from build123d import *

# Parameters (mm, degrees)
SALIENTE_EXTRUIR1_DEPTH = 3
CROQUIS3_W              = 30
CROQUIS3_H              = 10
CORTAR_EXTRUIR1_DEPTH   = 4


with BuildPart() as part:
    # Croquis2 → Saliente-Extruir1 (new body)
    with BuildSketch(Plane(origin=(0, 0, 0), x_dir=(0, 0, -1), z_dir=(1, 0, 0))):
        Polygon((-16.25, 20), (16.25, 20), (32.25, -45), (-32.25, -45), align=None)
    extrude(amount=SALIENTE_EXTRUIR1_DEPTH)

    # Croquis3 → Cortar-Extruir1 (cut, through all)
    with BuildSketch(Plane(origin=(3, 0, 0), x_dir=(0, 0, -1), z_dir=(1, 0, 0))):
        with Locations((0, -5)):
            Rectangle(CROQUIS3_W, CROQUIS3_H)
    extrude(amount=-CORTAR_EXTRUIR1_DEPTH, mode=Mode.SUBTRACT)


solid = part.part
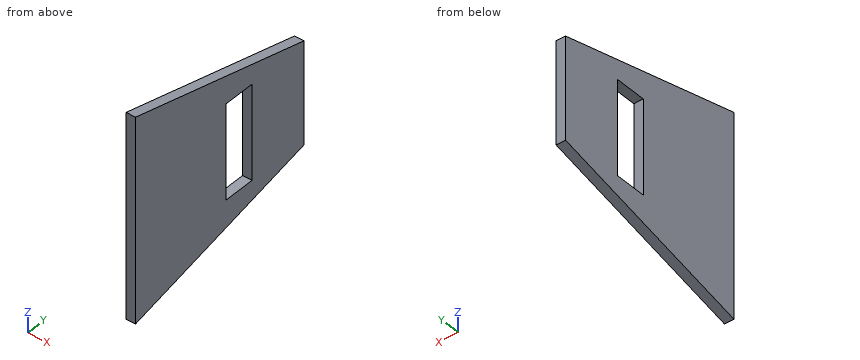
Part model, mm, in its own coordinate system. Round coordinates to 2 decimals unless told otherwise and drop trailing zeros. Loops run counter-clockwise (first coordinate to the right, second up) from the corner with the lowest first, then second, coordinate; pieces in that order, holes last. Notation, with made-up numbers: (4, 62.25) - (58, 62.25) arc R11 ccw to (58, 81.25) - close; hole circle Ø1 at (36, 13). An arc over 180 degrees is marked (long way). Answer as a JSON object with one key per item and string values.
Item 1: Band-saw the part on D-D on y = -24. List the corners of the cut face in (x, z).
Output:
{"outline": "(0, -27.08) - (3, -27.08) - (3, 27.08) - (0, 27.08) - close"}
Item 2: Wall check: L1, parallel to Y at x = 2.4, z = -5.5; L2, parallel to Z at x = 2.2, y = -2; L3, parallel to Z at x = 0.55, y = -1. Give the ranges that are in metal, low to high.
Output:
{"L1": "-45 to -10, 0 to 20", "L2": "-21.67 to -15, 15 to 21.67", "L3": "-21.42 to -15, 15 to 21.42"}
Item 3: Band-saw the part on C-C on x = 0.75. List the corners of the cut face in (y, z).
Output:
{"outline": "(-45, -32.25) - (20, -16.25) - (20, 16.25) - (-45, 32.25) - close; hole (-10, -15) - (0, -15) - (0, 15) - (-10, 15) - close"}
Item 4: Pin check, flat tips, straight feed: pin 1 (1.5 mm diameter, centred on x = 0.5, y = 2.5, fed in from -Z); pin 2 (1.5 mm diameter, centred on x = 1.5, y = -6.5, fed in from -Z). Stop position of each tip, or through.
Output:
{"pin 1": "z = -20.74", "pin 2": "z = -22.96"}
Item 5: Band-saw the part on B-B on y = -1. List the corners of the cut face in (x, z).
Output:
{"outline": "(0, -21.42) - (3, -21.42) - (3, -15) - (0, -15) - close; (0, 15) - (3, 15) - (3, 21.42) - (0, 21.42) - close"}
Item 6: Band-saw the part on A-A on z = 1. List the corners of the cut face in (x, y).
Output:
{"outline": "(0, -45) - (3, -45) - (3, -10) - (0, -10) - close; (0, 0) - (3, 0) - (3, 20) - (0, 20) - close"}
